Autodesk Fusion 360 part; units mm, degrees
sketch "Sketch1" plane through (0, 0, 0) normal (0, 0, 1) x (1, 0, 0)
  circle A0 centre (0, 0) radius 6
  line L0 (0, 0) -> (0, 49.4759) construction
  line L1 (0, 0) -> (0, -54.6862) construction
  arc A1 (0, 18) -> (0, -18) centre (0, 0) ccw
  line L2 (0, 18) -> (25, 18)
  line L3 (0, -18) -> (25, -18)
  line L4 (25, 18) -> (25, -18)
  dimension "d1" = 36
  dimension "d2" = 12
  dimension "d4" = 25
  dimension "d5" = 25
extrude "Extrude1" add sketch "Sketch1" along normal mid plane 30
sketch "Sketch2" plane through (25, 0, 0) normal (1, 0, 0) x (0, 0, -1)
  line L0 (15, 18) -> (-15, 18)
  line L1 (-15, 18) -> (-15, -18)
  line L2 (-15, -18) -> (15, -18)
  line L3 (15, -18) -> (15, 18)
  circle A0 centre (0, 0) radius 19
  circle A1 centre (0, 0) radius 17
  dimension "d8" = 38
  dimension "d9" = 34
extrude "Extrude2" add sketch "Sketch2" along normal blind 1500 contours L0 L1 L3 A0 A1 | L0 A0 | L3 A0 A1 | L1 A0 A1 | L1 L2 L3 A0 A1 | L2 A0
ref_plane "WorkPlane1" through (25, 0, 0) normal (1, 0, 0) x (0, 1, 0)
sketch "Sketch3" plane through (25, 0, 0) normal (1, 0, 0) x (0, 0, -1)
  line L0 (-6.0828, 18) -> (-15, 18)
  line L1 (-15, 11.6619) -> (-15, 18)
  line L2 (15, 18) -> (6.0828, 18)
  line L3 (15, 18) -> (15, 11.6619)
  line L4 (-6.0828, -18) -> (-15, -18)
  line L5 (-15, -18) -> (-15, -11.6619)
  line L6 (15, -18) -> (6.0828, -18)
  line L7 (15, -11.6619) -> (15, -18)
  circle A0 centre (0, 0) radius 23.4307
extrude "Extrude3" add sketch "Sketch3" along normal mid plane 5
fillet "Fillet1" radius 5 4 edges at (22.5, 18, 0) (22.5, 0, 15) (22.5, -18, 0) (22.5, 0, -15)
sketch "Sketch4" plane through (0, 0, 0) normal (0, 1, 0) x (1, 0, 0)
  line L0 (0, 0) -> (50, 0) construction
  circle A0 centre (50, 0) radius 2.5
  dimension "d16" = 50
  dimension "d17" = 5
extrude "Extrude4" cut sketch "Sketch4" along normal through all and the other way through all
sketch "Sketch5" plane through (0, 0, 0) normal (0, 0, 1) x (1, 0, 0)
  line L0 (0, 0) -> (50, 0) construction
  circle A0 centre (50, 0) radius 2.5
  dimension "d20" = 50
  dimension "d21" = 5
extrude "Extrude5" cut sketch "Sketch5" along normal through all and the other way through all
equation "d1 = ( 18 * 2 ) * 1 mm"
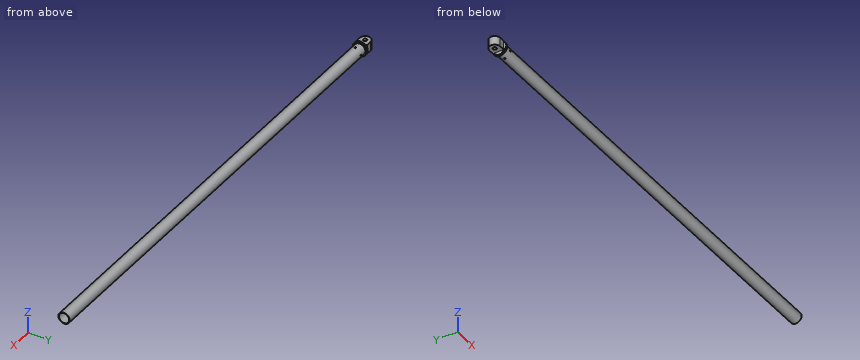
The model under review builds one solid part; all positions refer to its coordinate system, in mm. Round coordinates to 2 decimals unless told otherwise and drop trailing zeros. Loops run counter-clockwise (first coordinate to the right, second up) from the corner with the lowest first, then second, coordinate; pieces in that order, holes last.
1) Wall thickness on line 1 along X through (y, z) = (0, -17.75); line 2 along Z through (x, y) = (1235, -8.5); line 3 along X through (y, z) = (0, 17.7): over which ranges is each line inside the solid? List them lowest first.
Values follow:
line 1: x = 21.97 to 47.5, 52.5 to 1525
line 2: z = -16.99 to -14.72, 14.72 to 16.99
line 3: x = 21.94 to 47.5, 52.5 to 1525
2) Consider section A-A on x = 535.5. State the section outline as (y, z) points.
Values follow:
outline: circle Ø38 at (0, 0); hole circle Ø34 at (0, 0)
3) Clearance check with flat-ended pins moving along their axes: P1, Ø2, axis at x = 259, z = 17.5, coming from the +Y side; P2, Ø18, axis at x = 5.5, y = -2.5, coming from the +Z side; P3, Ø5, axis at y = 4.5, z = -4.5, coming from the -X side. State where each tip first meets the part, or that it passes through.
Values follow:
P1: stops at y = 9.42
P2: stops at z = 15
P3: stops at x = -17.89
